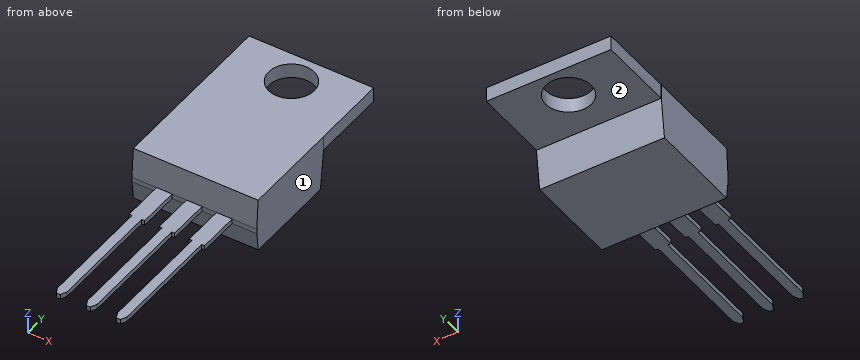
from build123d import *
from OCP.BRepFilletAPI import BRepFilletAPI_MakeChamfer

# Parameters (mm, degrees)
LINEAR_AUSTRAGEN1_DEPTH              = 5.2
F_3_8_3_8_DURCHMESSER_BOHRUNG1_D     = 3.8
F_3_8_3_8_DURCHMESSER_BOHRUNG1_DEPTH = 5
F_3_8_3_8_DURCHMESSER_BOHRUNG1_TIP   = 1.141635176
SKIZZE4_W                            = 1.3
SKIZZE4_H                            = 0.4
LINEAR_AUSTRAGEN2_DEPTH              = 3.5
SKIZZE5_W                            = 0.8
SKIZZE5_H                            = 0.4
LINEAR_AUSTRAGEN3_DEPTH              = 10
FASE1_SIZE                           = 0.5
FASE1_SIZE2                          = 0.233153829
SKIZZE7_W                            = 1.22
SKIZZE7_H                            = 6.4
SCHNITT_LINEAR_AUSTRAGEN1_DEPTH      = 0.01


with BuildPart() as part:
    # Skizze1 → Linear austragen1 (new, symmetric)
    with BuildSketch(Plane(origin=(0, 0, 0), x_dir=(0, 0, -1), z_dir=(1, 0, 0))):
        Polygon((0, 0), (1.22, 0), (1.22, -6.4), (4.499948007, -6.802726976), (4.499948007, -14.703551087), (2.9, -14.9), (2.5, -14.9), (0, -14.72518297), align=None)
    extrude(amount=LINEAR_AUSTRAGEN1_DEPTH, both=True)

    # Ø3.8 (3.8) Durchmesser Bohrung1
    with Locations(Plane(origin=(0, 0, -1.22), x_dir=(-1, 0, 0), z_dir=(0, 0, -1))):
        with Locations((0, -2.54)):
            Hole(F_3_8_3_8_DURCHMESSER_BOHRUNG1_D / 2, depth=F_3_8_3_8_DURCHMESSER_BOHRUNG1_DEPTH)
            with Locations((0, 0, -(F_3_8_3_8_DURCHMESSER_BOHRUNG1_DEPTH + F_3_8_3_8_DURCHMESSER_BOHRUNG1_TIP / 2))):  # 118° drill point
                Cone(0, F_3_8_3_8_DURCHMESSER_BOHRUNG1_D / 2, F_3_8_3_8_DURCHMESSER_BOHRUNG1_TIP, mode=Mode.SUBTRACT)

    # Skizze4 → Linear austragen2 (add)
    with BuildSketch(Plane.XZ.offset(14.9)):
        with Locations((-2.5, -2.7)):
            Rectangle(SKIZZE4_W, SKIZZE4_H)
        with Locations((0, -2.7)):
            Rectangle(SKIZZE4_W, SKIZZE4_H)
        with Locations((2.5, -2.7)):
            Rectangle(SKIZZE4_W, SKIZZE4_H)
    extrude(amount=LINEAR_AUSTRAGEN2_DEPTH)

    # Skizze5 → Linear austragen3 (add)
    with BuildSketch(Plane.XZ.offset(18.4)):
        with Locations((2.5, -2.7)):
            Rectangle(SKIZZE5_W, SKIZZE5_H)
        with Locations((0, -2.7)):
            Rectangle(SKIZZE5_W, SKIZZE5_H)
        with Locations((-2.5, -2.7)):
            Rectangle(SKIZZE5_W, SKIZZE5_H)
    extrude(amount=LINEAR_AUSTRAGEN3_DEPTH)

    # Fase1: one chamfer whose edges measure the first distance from different faces: ONE call of the kernel's chamfer builder (chamfer() names one face for all edges)
    fase1_edges_1 = [part.edges().sort_by_distance(p)[0] for p in [
        (-2.9, -28.4, -2.7),
    ]]
    fase1_side_1 = [part.faces().sort_by_distance(p)[0] for p in [
        (-2.9, -23.4, -2.7),
    ]]
    fase1_edges_2 = [part.edges().sort_by_distance(p)[0] for p in [
        (-2.1, -28.4, -2.7),
    ]]
    fase1_side_2 = [part.faces().sort_by_distance(p)[0] for p in [
        (-2.1, -23.4, -2.7),
    ]]
    fase1_edges_3 = [part.edges().sort_by_distance(p)[0] for p in [
        (0.4, -28.4, -2.7),
    ]]
    fase1_side_3 = [part.faces().sort_by_distance(p)[0] for p in [
        (0.4, -23.4, -2.7),
    ]]
    fase1_edges_4 = [part.edges().sort_by_distance(p)[0] for p in [
        (-0.4, -28.4, -2.7),
    ]]
    fase1_side_4 = [part.faces().sort_by_distance(p)[0] for p in [
        (-0.4, -23.4, -2.7),
    ]]
    fase1_edges_5 = [part.edges().sort_by_distance(p)[0] for p in [
        (2.1, -28.4, -2.7),
    ]]
    fase1_side_5 = [part.faces().sort_by_distance(p)[0] for p in [
        (2.1, -23.4, -2.7),
    ]]
    fase1_edges_6 = [part.edges().sort_by_distance(p)[0] for p in [
        (2.9, -28.4, -2.7),
    ]]
    fase1_side_6 = [part.faces().sort_by_distance(p)[0] for p in [
        (2.9, -23.4, -2.7),
    ]]
    fase1 = BRepFilletAPI_MakeChamfer(part.part.solid().wrapped)
    for e in fase1_edges_1:
        fase1.Add(FASE1_SIZE, FASE1_SIZE2, e.wrapped, fase1_side_1[0].wrapped)  # the first distance lies on this face
    for e in fase1_edges_2:
        fase1.Add(FASE1_SIZE, FASE1_SIZE2, e.wrapped, fase1_side_2[0].wrapped)  # the first distance lies on this face
    for e in fase1_edges_3:
        fase1.Add(FASE1_SIZE, FASE1_SIZE2, e.wrapped, fase1_side_3[0].wrapped)  # the first distance lies on this face
    for e in fase1_edges_4:
        fase1.Add(FASE1_SIZE, FASE1_SIZE2, e.wrapped, fase1_side_4[0].wrapped)  # the first distance lies on this face
    for e in fase1_edges_5:
        fase1.Add(FASE1_SIZE, FASE1_SIZE2, e.wrapped, fase1_side_5[0].wrapped)  # the first distance lies on this face
    for e in fase1_edges_6:
        fase1.Add(FASE1_SIZE, FASE1_SIZE2, e.wrapped, fase1_side_6[0].wrapped)  # the first distance lies on this face
    add(Compound.cast(fase1.Shape()), mode=Mode.REPLACE)

    # Skizze7 → Schnitt-Linear austragen1 (cut)
    with BuildSketch(Plane.ZY.offset(5.2)):
        with Locations((-0.61, -3.2)):
            Rectangle(SKIZZE7_W, SKIZZE7_H)
    schnitt_linear_austragen1 = extrude(amount=-SCHNITT_LINEAR_AUSTRAGEN1_DEPTH, mode=Mode.SUBTRACT)

    # Spiegeln1: Schnitt-Linear austragen1 across plane
    add(schnitt_linear_austragen1.mirror(Plane(origin=(0, 0, 0), x_dir=(0, 0, 1), z_dir=(1, 0, 0))), mode=Mode.SUBTRACT)


solid = part.part
Input: part model. Units: mm. Frame: model coordinates. Face numbers are marked on the shaded views. A direction names the side the tool comes from. Give positions to 0.01 mm unless a question says otherwise; leave off trailing zeros. Order: outer loops, then holes, each group sorted by start corner. A loop starts at its lowest first (then second) coordinate and runs counter-clockwise, first axis right, second up. Notation, with made-up numbers: (-29, 30.5) - (10, 30.5) arc R28 ccw to (10, 48.5) - close; hole circle Ø5 at (42.25, 15). An arc over 180 degrees is marked (long way). Answer as a JSON object with one key per item and string values. Group by question number.
Q1. Cut plane D-D, the plane y = -16.5. Output: boundary loops of the cut face in (x, z).
Q2. Set-up query: the marked faces 1 and 2. Return all of +Z, -Z, +X, -X, +Y, -Y with unobstructed straight access to the full face (end or side cutting, diameter ignored); none if empty.
Q3. First-contact query: pin 1 Ø1 at (x, z) = (1.5, -1.5) entering from +Y; pin 2 Ø1 at (x, y) = (-2.5, -20.5) entering from -Z; pin 3 Ø1.5 at (y, z) = (-19, -0.5) entering from +X; pin 4 Ø1.4 at (x, y) = (-3, -23) entering from +Z. Flat tips, straight axial feed; report the tip coordinate or a pass-through.
Q4. Cut plane B-B, the plane y = -22.75. Output: boundary loops of the cut face in (x, z).
Q5. Cut plane A-A, the plane y = -2.54. Output: boundary loops of the cut face in (x, z).
Q6. Cut plane C-C, the plane x = -4.5. Output: boundary loops of the cut face in (y, z), then the cut area to 3 significant figures.
Q7. Line query: probe 1 along Z at (x, y) = (0, -15.5); probe 2 along Y at (x, z) = (0, -0.7); probe 3 along Y at (x, z) = (0, -0.25). Output: solid intervals per line, ascending.
Results:
{
 "1": {"outline": "(-3.15, -2.9) - (-1.85, -2.9) - (-1.85, -2.5) - (-3.15, -2.5) - close; (-0.65, -2.9) - (0.65, -2.9) - (0.65, -2.5) - (-0.65, -2.5) - close; (1.85, -2.9) - (3.15, -2.9) - (3.15, -2.5) - (1.85, -2.5) - close"},
 "2": {"face 1": "+Z, -Z, +X, +Y, -Y", "face 2": "-Z, +X, -X, +Y"},
 "3": {"pin 1": "y = 0", "pin 2": "z = -2.9", "pin 3": "through", "pin 4": "z = -2.5"},
 "4": {"outline": "(-2.9, -2.9) - (-2.1, -2.9) - (-2.1, -2.5) - (-2.9, -2.5) - close; (-0.4, -2.9) - (0.4, -2.9) - (0.4, -2.5) - (-0.4, -2.5) - close; (2.1, -2.9) - (2.9, -2.9) - (2.9, -2.5) - (2.1, -2.5) - close"},
 "5": {"outline": "(-5.19, -1.22) - (-1.9, -1.22) - (-1.9, 0) - (-5.19, 0) - close; (1.9, -1.22) - (5.19, -1.22) - (5.19, 0) - (1.9, 0) - close"},
 "6": {"outline": "(-14.9, -2.9) - (-14.7, -4.5) - (-6.8, -4.5) - (-6.4, -1.22) - (0, -1.22) - (0, 0) - (-14.73, 0) - (-14.9, -2.5) - close", "area": "45.0 mm^2"},
 "7": {"probe 1": "-2.9 to -2.5", "probe 2": "-14.77 to -4.44, -0.64 to 0", "probe 3": "-14.74 to -4.44, -0.64 to 0"}
}
